Design review of the part built by this model. Coordinates are the model's own, in mm. A direction names the side the tool comes from. Coordinates: 2 decimals unless noted, no trailing zeros. Order: outer loops, then holes, each group sorted by start corner. A loop starts at its lowest first (then second) coordinate and runs counter-clockwise, first axis right, second up. Notation, with made-up numbers: M -34.5,-18.75 L -12.5,-18.75 A16 ccw -12.5,-14.75 Z; hole C 79.5,-22.5 d5. An arc over 180 degrees is marked long. Answer in a Markdown table with one row per item.
from build123d import *

# Parameters (mm, degrees)
SKETCH1_R               = 17.175
BOSS_EXTRUDE2_DEPTH     = 25
SHELL1_T                = -3.175
SKETCH3_R               = 3
CUT_EXTRUDE1_DEPTH      = 35.856294267
CUT_EXTRUDE1_DEPTH_BACK = 35.856294267
SKETCH5_R               = 2
BOSS_EXTRUDE3_DEPTH     = 5
FILLET1_R               = 1


with BuildPart() as part:
    # Sketch1 → Boss-Extrude2 (new body)
    with BuildSketch(Plane(origin=(0, 0, 0), x_dir=(1, 0, 0), z_dir=(0, 1, 0))):
        with Locations(Location((0, 0, 0), (0, 0, 270))):
            Circle(SKETCH1_R)
    extrude(amount=BOSS_EXTRUDE2_DEPTH)

    # Shell1
    shell1_openings = [part.faces().sort_by_distance(p)[0] for p in [
        (0, 0, 0),
    ]]
    offset(amount=SHELL1_T, openings=shell1_openings, kind=Kind.INTERSECTION)

    # Sketch3 → Cut-Extrude1 (cut, two sides)
    with BuildSketch(Plane(origin=(0, 0, 0), x_dir=(0, 0, -1), z_dir=(1, 0, 0))) as cut_extrude1_sk:
        with Locations((0, 12.5)):
            Circle(SKETCH3_R)
    extrude(amount=CUT_EXTRUDE1_DEPTH, mode=Mode.SUBTRACT)
    extrude(cut_extrude1_sk.sketch, amount=-CUT_EXTRUDE1_DEPTH_BACK, mode=Mode.SUBTRACT)

    # Sketch5 → Boss-Extrude3 (add, symmetric)
    with BuildSketch(Plane(origin=(0, 0, 0), x_dir=(0, 0, -1), z_dir=(1, 0, 0))):
        with BuildLine():
            Line((-10, 36), (-10, 25))
            Line((-10, 25), (-10, 24.25))
            Line((-10, 24.25), (10, 24.25))
            Line((10, 24.25), (10, 25))
            Line((10, 25), (10, 36))
            ThreePointArc((10, 36), (0, 46), (-10, 36))
        make_face()
        with Locations((0, 36)):
            Circle(SKETCH5_R, mode=Mode.SUBTRACT)
    extrude(amount=BOSS_EXTRUDE3_DEPTH, both=True)

    # Fillet1
    fillet1_edges = [part.edges().sort_by_distance(p)[0] for p in [
        (0, 25, -17.175),
    ]]
    fillet(fillet1_edges, radius=FILLET1_R)


solid = part.part
(1) Add section A-A, the plane z = 0. Give the boundary of the cut face in (x, y) (3 decimals), and give its area (3 significant figures).
Return value:
| item | result |
|---|---|
| outline | M -17.175,0 L -14,0 L -14,9.5 L -17.175,9.5 Z; M -17.175,15.5 L -14,15.5 L -14,21.825 L 14,21.825 L 14,15.5 L 17.175,15.5 L 17.175,24 A1 ccw 16.175,25 L 5,25 L 5,34 L -5,34 L -5,25 L -16.175,25 A1 ccw -17.175,24 Z; M -5,38 L 5,38 L 5,46 L -5,46 Z; M 14,0 L 17.175,0 L 17.175,9.5 L 14,9.5 Z |
| area | 379 mm2 |
(2) Insertion check: pin 1 Ø11 at (x, y) = (-0.5, 31.5) entering from +Z; pin 2 Ø3.5 at (y, z) = (36, 0) entering from -X; pin 3 Ø16 at (y, z) = (38, -4.5) entering from +X; pin 4 Ø4 at (y, z) = (11.5, 2.5) entering from -X. Each pin has a flat end and moves straight along its axis. Give the tip position at first contact, or say it passes through.
Return value:
| item | result |
|---|---|
| pin 1 | stops at z = 10 |
| pin 2 | passes through |
| pin 3 | stops at x = 5 |
| pin 4 | stops at x = -17.12 |
(3) For faces 1 (the cylindrical face through (15.4, 12.6, 3)), 2 (the cylindrical face through (-12.4, 10.8, 6.5)), 3 (the flat face through (5, 33, 0)), 4 (the flat face through (0, 30, -10)), 5 (the flat face through (-5, 33, 0)), list the 3-axis set-ups (+Z, -Z, +X, -X, +Y, -Y) from which the entire face can be reached by the end or side of a thin tool; tool diameter is ignored.
Return value:
| item | result |
|---|---|
| face 1 | +X, -X |
| face 2 | -Y |
| face 3 | +Z, -Z, +X, +Y |
| face 4 | -Z, +X, -X, +Y |
| face 5 | +Z, -Z, -X, +Y |
(4) Add section B-B, the plane x = 0. Give the boundary of the cut face in (y, z) (3 decimals), and give its area (3 significant figures).
Return value:
| item | result |
|---|---|
| outline | M 0,-17.175 L 24,-17.175 A1 ccw 25,-16.175 L 25,-10 L 36,-10 A10 ccw 36,10 L 25,10 L 25,16.175 A1 ccw 24,17.175 L 0,17.175 L 0,14 L 21.825,14 L 21.825,-14 L 0,-14 Z; hole C 36,0 d4 |
| area | 612 mm2 |
(5) For line 1 along Y through (x, z) = (-1, 0) (3 decimals); line 2 along Y through (x, z) = (15, 0); line 3 along X through (y, z) = (25.5, 2), list the stretches that pass through material, from the lowest coordinate up. Write a range as from..to.
Return value:
| item | result |
|---|---|
| line 1 | y = 21.825..34, 38..46 |
| line 2 | y = 0..9.5, 15.5..25 |
| line 3 | x = -5..5 |
(6) Draft analysis for pull direction Y (two halves, no side actions). For faces 6 (the flat face through (0, 31, 10)), 7 (the cylindrical face through (-15.4, 12.6, 3)), 8 (the flat face through (-13, 0, -6)), 9 (the cylindrical face through (0, 34, 0)), state which applies: pulls with the +Y half, pulls with the -Y half, needs draft (parallel to the pull), parting line crosses it, or undercut.
Return value:
| item | result |
|---|---|
| face 6 | needs draft |
| face 7 | undercut |
| face 8 | pulls with the -Y half |
| face 9 | undercut |
